CAD build for the part. Positions are in the model's coordinates, mm. Face numbers are marked on the shaded views. Give positions to 0.01 mm unless a question says otherwise; leave off trailing zeros. Write each loop counter-clockwise with the first axis right and the second up, starting at its lowest first coordinate (ties: lowest second). Pieces come first, ordered by that corner, then holes. Notation, with made-up numbers: (73.5, 86.5) -> (91.5, 86.5) arc R22 cw to (91.5, 121.5) -> close; hole circle Ø11 at (3.5, -24.75). An arc over 180 degrees is marked (long way). Use one line per item in the form item = value. Start each with the question number.
from build123d import *

# Parameters (mm, degrees)
F0_R     = 19.05
F0_R_2   = 12.7
F0_R_3   = 6.35
F1_DEPTH = 6.858
F2_T     = -2.54


# Not quite as in the source:
# - a fillet or chamfer that OpenCascade refuses, or shapes differently, is made with other operations: its cross-section is extruded or revolved along the edge and cut away or added
# - the program builds the solid bodies; features that only make, move or delete a surface that nothing else refers to are left out


with BuildPart() as f1:
    # F0 (on Right) → F1 (new body, symmetric)
    with BuildSketch(Plane.YZ):
        Circle(F0_R)
        Circle(F0_R_2, mode=Mode.SUBTRACT)
        Circle(F0_R_2)
        Circle(F0_R_3, mode=Mode.SUBTRACT)
        Circle(F0_R_3)
    extrude(amount=F1_DEPTH, both=True)

    # F2
    f2_openings = [f1.faces().sort_by_distance(p)[0] for p in [
        (6.858, 0, 0),
    ]]
    offset(amount=F2_T, openings=f2_openings)

    # F4: fillet of radius 4.9056819587 on 1 edges, made by hand

    # F4_s1 → F4_t2 (revolve, cut)
    with BuildSketch(Plane.XY):
        with BuildLine():
            ThreePointArc((6.858, 19.05), (5.0564518797, 17.1924723508), (2.5604117984, 16.51))
            Line((2.5604117984, 16.51), (6.858, 16.51))
            Line((6.858, 16.51), (6.858, 19.05))
        make_face()
    revolve(axis=Axis((6.858, 0, 0), (1, 0, 0)), mode=Mode.SUBTRACT)


solid = f1.part
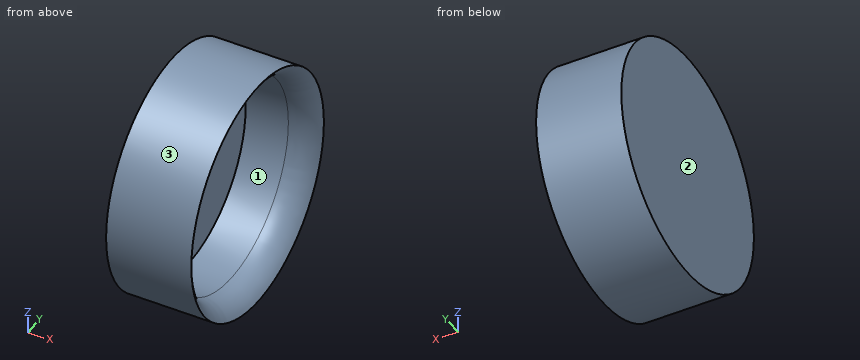
1) Pin check, flat tips, straight feed: pin 1 (1.5 mm diameter, centred on x = -5, y = 3.5, fed in from +Z); pin 2 (4 mm diameter, centred on x = -4, z = 3.5, fed in from +Y); pin 3 (10 mm diameter, centred on y = 1, z = 4.5, fed in from +X). Stop position of each tip, or through.
2) Cut at D-D (x = -5.25). Give the cut face in (y, z).
3) Wall check: line 1 along Z through (x, y) = (0, 0); line 2 along X through (y, z) = (-3.5, -14); line 3 along Z through (x, y) = (0.25, 12). Give the ranges that are in metal, low to high. Write a range as from..to.
4) Two-plate mould, pull along Z, no slides. Class the marked faces 1, 2 and 3: released by +Z, released by -Z, zero draft, split by the parting line, or undercut.
5) Cut at C-C (x = -1.75). Give the cut face in (y, z), and give its area (3 significant figures).
6) Cut at A-A (z = 0). Give the cut face in (x, y), and give its area (3 significant figures).
Final values:
q1.pin_1 = 18.85
q1.pin_2 = 18.99
q1.pin_3 = -4.32
q2.outline = circle Ø38.1 at (0, 0)
q3.line_1 = -19.05..-16.51, 16.51..19.05
q3.line_2 = -6.86..-4.32
q3.line_3 = -14.8..-11.34, 11.34..14.8
q4.face_1 = undercut
q4.face_2 = zero draft
q4.face_3 = split by the parting line
q5.outline = circle Ø38.1 at (0, 0); hole circle Ø33.02 at (0, 0)
q5.area = 284 mm^2
q6.outline = (-6.86, -19.05) -> (6.86, -19.05) arc R4.91 ccw to (2.56, -16.51) -> (-4.32, -16.51) -> (-4.32, 16.51) -> (2.56, 16.51) arc R4.91 ccw to (6.86, 19.05) -> (-6.86, 19.05) -> close
q6.area = 147 mm^2
